The listing builds one solid part. Answer for the finished solid, in the listing's coordinates (mm). A direction names the side the tool comes from. Coordinates: 2 decimals unless noted, no trailing zeros. Order: outer loops, then holes, each group sorted by start corner. A loop starts at its lowest first (then second) coordinate and runs counter-clockwise, first axis right, second up.
from build123d import *
from build123d.topology import SkipClean

# Parameters (mm, degrees)
SALIENTE_EXTRUIR2_DEPTH    = 70
SALIENTE_EXTRUIR4_START    = -4
SALIENTE_EXTRUIR4_DEPTH    = 4
SALIENTE_EXTRUIR5_START    = 70
SALIENTE_EXTRUIR5_DEPTH    = 4
CORTAR_EXTRUIR1_DEPTH      = 15
CORTAR_EXTRUIR1_DEPTH_BACK = 79.568441502
CROQUIS5_RX                = 30
CROQUIS5_RY                = 5.809368516
SALIENTE_EXTRUIR6_DEPTH    = 50
CROQUIS7_W                 = 2
CROQUIS7_H                 = 74
SALIENTE_EXTRUIR7_DEPTH    = 15.745948
CROQUIS9_R                 = 2.65
CROQUIS9_W                 = 11
CROQUIS9_H                 = 6
CORTAR_EXTRUIR2_DEPTH      = 10
CORTAR_EXTRUIR3_REACH      = 100.697
CROQUIS10_W                = 13.5
CROQUIS10_H                = 9


with BuildPart() as part:
    # Croquis1 → Saliente-Extruir2 (new body)
    with BuildSketch(Plane.XY):
        with BuildLine():
            Line((-9, 6.745948294), (-7.15808144, 6.745948294))
            ThreePointArc((-7.15808144, 6.745948294), (-6.702907265, 6.452869704), (-6.781340312, 5.917214173))
            ThreePointArc((-6.781340312, 5.917214173), (0, -9), (6.781340312, 5.917214173))
            ThreePointArc((6.781340312, 5.917214173), (6.702907265, 6.452869704), (7.15808144, 6.745948294))
            Line((7.15808144, 6.745948294), (9, 6.745948294))
            ThreePointArc((9, 6.745948294), (11.121320344, 5.867268638), (12, 3.745948294))
            Line((12, 3.745948294), (12, -11))
            Line((12, -11), (-12, -11))
            Line((-12, -11), (-12, 3.745948294))
            ThreePointArc((-12, 3.745948294), (-11.121320344, 5.867268638), (-9, 6.745948294))
        make_face()
    extrude(amount=SALIENTE_EXTRUIR2_DEPTH)

    # Croquis1<6> → Saliente-Extruir4 (add)
    with BuildSketch(Plane.XY.offset(SALIENTE_EXTRUIR4_START)):
        with BuildLine():
            Line((7.15808144, 6.745948294), (9, 6.745948294))
            ThreePointArc((9, 6.745948294), (11.121320344, 5.867268638), (12, 3.745948294))
            Line((12, 3.745948294), (12, -11))
            Line((12, -11), (-12, -11))
            Line((-12, -11), (-12, 3.745948294))
            ThreePointArc((-12, 3.745948294), (-11.121320344, 5.867268638), (-9, 6.745948294))
            Line((-9, 6.745948294), (-7.15808144, 6.745948294))
            ThreePointArc((-7.15808144, 6.745948294), (-6.702907265, 6.452869704), (-6.781340312, 5.917214173))
            ThreePointArc((-6.781340312, 5.917214173), (0, -9), (6.781340312, 5.917214173))
            ThreePointArc((6.781340312, 5.917214173), (6.702907265, 6.452869704), (7.15808144, 6.745948294))
        make_face()
        with BuildLine():
            Line((7.15808144, 6.745948294), (-7.15808144, 6.745948294))
            ThreePointArc((-7.15808144, 6.745948294), (-6.702907265, 6.452869704), (-6.781340312, 5.917214173))
            ThreePointArc((-6.781340312, 5.917214173), (0, -9), (6.781340312, 5.917214173))
            ThreePointArc((6.781340312, 5.917214173), (6.702907265, 6.452869704), (7.15808144, 6.745948294))
        make_face()
    extrude(amount=SALIENTE_EXTRUIR4_DEPTH)

    # Croquis1<9> → Saliente-Extruir5 (add)
    with BuildSketch(Plane.XY.offset(SALIENTE_EXTRUIR5_START)):
        with BuildLine():
            Line((7.15808144, 6.745948294), (9, 6.745948294))
            ThreePointArc((9, 6.745948294), (11.121320344, 5.867268638), (12, 3.745948294))
            Line((12, 3.745948294), (12, -11))
            Line((12, -11), (-12, -11))
            Line((-12, -11), (-12, 3.745948294))
            ThreePointArc((-12, 3.745948294), (-11.121320344, 5.867268638), (-9, 6.745948294))
            Line((-9, 6.745948294), (-7.15808144, 6.745948294))
            ThreePointArc((-7.15808144, 6.745948294), (-6.702907265, 6.452869704), (-6.781340312, 5.917214173))
            ThreePointArc((-6.781340312, 5.917214173), (0, -9), (6.781340312, 5.917214173))
            ThreePointArc((6.781340312, 5.917214173), (6.702907265, 6.452869704), (7.15808144, 6.745948294))
        make_face()
        with BuildLine():
            Line((7.15808144, 6.745948294), (-7.15808144, 6.745948294))
            ThreePointArc((-7.15808144, 6.745948294), (-6.702907265, 6.452869704), (-6.781340312, 5.917214173))
            ThreePointArc((-6.781340312, 5.917214173), (0, -9), (6.781340312, 5.917214173))
            ThreePointArc((6.781340312, 5.917214173), (6.702907265, 6.452869704), (7.15808144, 6.745948294))
        make_face()
    extrude(amount=SALIENTE_EXTRUIR5_DEPTH)

    # Croquis5 → Cortar-Extruir1 (cut, two sides: drawn at the far end of the back side and taken through both)
    with BuildSketch(Plane(origin=(12, 0, 0), x_dir=(0, 0, -1), z_dir=(1, 0, 0)).offset(-CORTAR_EXTRUIR1_DEPTH_BACK)):
        with Locations(Location((-35, 6.745948294), (0, 0, 0))):
            Ellipse(CROQUIS5_RX, CROQUIS5_RY)
        Polygon((0, 5.917214173), (0, -9), (-0.999510264, -9), (-0.999510264, 5.948506852), (-0.999510264, 6.745948294), (0, 6.745948294), align=None)
        Polygon((-70, 5.917214173), (-70, -9), (-69.000489736, -9), (-69.000489736, 5.948506852), (-69.000489736, 6.745948294), (-70, 6.745948294), align=None)
    extrude(amount=CORTAR_EXTRUIR1_DEPTH + CORTAR_EXTRUIR1_DEPTH_BACK, mode=Mode.SUBTRACT)

    # Croquis6 → Saliente-Extruir6 (add)
    with BuildSketch(Plane(origin=(12, 0, 0), x_dir=(0, 0, -1), z_dir=(1, 0, 0))):
        Polygon((-74, -11), (4, -11), (4, -9), (4, 6.745948294), (2, 6.745948294), (2, -9), (-72, -9), (-72, 6.745948294), (-74, 6.745948294), (-74, -9), align=None)
    extrude(amount=SALIENTE_EXTRUIR6_DEPTH)

    # Croquis7 → Saliente-Extruir7 (add)
    with SkipClean():  # the faces are left unmerged after this step: merging them gives an invalid solid
        with BuildSketch(Plane(origin=(0, -9, 0), x_dir=(1, 0, 0), z_dir=(0, 1, 0))):
            with Locations((61, -35)):
                Rectangle(CROQUIS7_W, CROQUIS7_H)
        extrude(amount=SALIENTE_EXTRUIR7_DEPTH)

    # Croquis9 → Cortar-Extruir2 (cut)
    with SkipClean():  # the faces are left unmerged after this step: merging them gives an invalid solid
        with BuildSketch(Plane(origin=(0, -9, 0), x_dir=(1, 0, 0), z_dir=(0, 1, 0))):
            with Locations(Location((51.5, -53.035506603, 0), (0, 0, 270))):
                Circle(CROQUIS9_R)
            with Locations((51.5, -35)):
                Rectangle(CROQUIS9_W, CROQUIS9_H)
        extrude(amount=-CORTAR_EXTRUIR2_DEPTH, mode=Mode.SUBTRACT)

    # Croquis10 → Cortar-Extruir3 (cut, up to next)
    with BuildSketch(Plane.XY.offset(-2), mode=Mode.PRIVATE) as cortar_extruir3_sk1:
        with Locations((25.297097726, 2.245948294)):
            Rectangle(CROQUIS10_W, CROQUIS10_H)
    cortar_extruir3_tool1 = extrude(cortar_extruir3_sk1.sketch, amount=-CORTAR_EXTRUIR3_REACH, mode=Mode.PRIVATE) & part.part
    add(cortar_extruir3_tool1.solids().sort_by_distance((25.297098, 2.245948, -2))[0], mode=Mode.SUBTRACT)


solid = part.part
1) Section A-A (y = 0) is taken. Give the vertices of the cut face in (x, z), then the cut area to 3 significant figures.
2) Section B-B (x = 38) is taken. Give the vertices of the cut face in (y, z).
3) Section D-D (x = 26.5) is taken. Give the vertices of the cut face in (y, z).
4) Consider L1, parallel to X at y = 0, z = 35; L2, parallel to Z at x = 10.5, y = -4; L3, parallel to Z at x = 56, y = -9.5. Determine where each line is inside the solid, lowest interval first.
5) Determine the mould class of faces 6 (the face through (-11.476, 5.44, 66.634)), 7 (the face through (36, -1, -2)), 8 (the face through (15, 6.746, -3)) for opening direction X: released by +X, released by -X, zero draft, split by the parting line, or undercut.
6) Section C-C (y = -5) is taken. Give the vertices of the cut face in (x, z), then the cut area to 3 significant figures.
7) A tool of negligible diameter and unlimited length cuts with its end or side. For faces 1 (the face through (51, -10, 38)), 2 (the face through (10, -2, 69)), 3 (the face through (12, -3, -1)), 4 (the face through (8, 6.746, 67)), 5 (the face through (32.047, 2, -3)), from which of +Z, -Z, +X, -X, +Y, -Y can it reach the whole face along a straight path? Write none if from no direction.
8) Each of these flat-tipped pins is pushed along its axis until it touches: P1, Ø21.5, axis at x = 16, z = 41, coming from the +Y side; P2, Ø1, axis at x = 53.5, z = 50, coming from the +Y side; P3, Ø1.6, axis at x = 24.5, z = -2.5, coming from the +Y side; P4, Ø4, axis at x = 51.5, z = 53.04, coming from the +Y side. Where does it stop, or does it pass through?
Filled sheet:
1. outline: (-12, -4) - (18.55, -4) - (18.55, -2) - (12, -2) - (12, 0) - (-12, 0) - close; (-12, 1) - (-9, 1) - (-9, 69) - (-12, 69) - close; (-12, 70) - (12, 70) - (12, 72) - (60, 72) - (60, -2) - (32.05, -2) - (32.05, -4) - (62, -4) - (62, 74) - (-12, 74) - close; (9, 1) - (12, 1) - (12, 69) - (9, 69) - close
1. area: 921 mm2
2. outline: (-11, -4) - (6.75, -4) - (6.75, -2) - (-9, -2) - (-9, 72) - (6.75, 72) - (6.75, 74) - (-11, 74) - close
3. outline: (-11, -4) - (-2.25, -4) - (-2.25, -2) - (-9, -2) - (-9, 72) - (6.75, 72) - (6.75, 74) - (-11, 74) - close
4. L1: x = -12 to -9, 9 to 12, 60 to 62
4. L2: z = -4 to 0, 1 to 69, 70 to 74
4. L3: z = -4 to 32, 38 to 74
5. face 6: released by -X
5. face 7: undercut
5. face 8: zero draft
6. outline: (-12, -4) - (62, -4) - (62, 74) - (-12, 74) - (-12, 70) - (12, 70) - (12, 72) - (60, 72) - (60, -2) - (12, -2) - (12, 0) - (-12, 0) - close; (-12, 1) - (-7.48, 1) - (-7.48, 69) - (-12, 69) - close; (7.48, 1) - (12, 1) - (12, 69) - (7.48, 69) - close
6. area: 1,150 mm2
7. face 1: +Y, -Y
7. face 2: -X, +Y
7. face 3: +Y
7. face 4: +Z, -Z, +X, -X, +Y
7. face 5: -Z, +Y
8. P1: stops at y = 1.83
8. P2: stops at y = -9
8. P3: stops at y = -2.25
8. P4: passes through
